```python
from build123d import *

# Parameters (mm, degrees)
SKETCH1_W           = 50
SKETCH1_H           = 70
SKETCH1_W_2         = 42
SKETCH1_H_2         = 62
BOSS_EXTRUDE2_DEPTH = 1400
SKETCH2_R           = 15
CUT_EXTRUDE1_DEPTH  = 1403.640367307


with BuildPart() as part:
    # Sketch1 → Boss-Extrude2 (new body)
    with BuildSketch(Plane.XY):
        with Locations((25, -35)):
            Rectangle(SKETCH1_W, SKETCH1_H)
        with Locations((25, -35)):
            Rectangle(SKETCH1_W_2, SKETCH1_H_2, mode=Mode.SUBTRACT)
    extrude(amount=BOSS_EXTRUDE2_DEPTH)

    # Sketch2 → Cut-Extrude1 (cut, through all)
    with BuildSketch(Plane(origin=(50, 0, 0), x_dir=(0, 0, -1), z_dir=(1, 0, 0))):
        with Locations(Location((-1050, -23, 0), (0, 0, 90))):
            Circle(SKETCH2_R)
        with Locations(Location((-200, -23, 0), (0, 0, 90))):
            Circle(SKETCH2_R)
        with Locations(Location((-810, -23, 0), (0, 0, 90))):
            Circle(SKETCH2_R)
        with Locations(Location((-360, -23, 0), (0, 0, 90))):
            Circle(SKETCH2_R)
        with BuildLine():
            Line((-1281.339745962, -30), (-1280, -30))
            ThreePointArc((-1280, -30), (-1275, -35), (-1280, -40))
            Line((-1280, -40), (-1281.339745962, -40))
            ThreePointArc((-1281.339745962, -40), (-1290, -45), (-1298.660254038, -40))
            Line((-1298.660254038, -40), (-1300, -40))
            ThreePointArc((-1300, -40), (-1305, -35), (-1300, -30))
            Line((-1300, -30), (-1298.660254038, -30))
            ThreePointArc((-1298.660254038, -30), (-1290, -25), (-1281.339745962, -30))
        make_face()
        with BuildLine():
            Line((-611.339745962, -30), (-610, -30))
            ThreePointArc((-610, -30), (-605, -35), (-610, -40))
            Line((-610, -40), (-611.339745962, -40))
            ThreePointArc((-611.339745962, -40), (-620, -45), (-628.660254038, -40))
            Line((-628.660254038, -40), (-630, -40))
            ThreePointArc((-630, -40), (-635, -35), (-630, -30))
            Line((-630, -30), (-628.660254038, -30))
            ThreePointArc((-628.660254038, -30), (-620, -25), (-611.339745962, -30))
        make_face()
    extrude(amount=-CUT_EXTRUDE1_DEPTH, mode=Mode.SUBTRACT)


solid = part.part
```
Part model, mm, in its own coordinate system. A direction names the side the tool comes from. Round coordinates to 2 decimals unless told otherwise and drop trailing zeros. Write each loop counter-clockwise with the first axis right and the second up, starting at its lowest first coordinate (ties: lowest second). Pieces come first, ordered by that corner, then holes. Notation, with made-up numbers: (73, 45.5) -> (115, 45.5) arc R25 cw to (115, 70.5) -> close; hole circle Ø3 at (55.5, 14). An arc over 180 degrees is marked (long way). Return JSON: item names as keys, results as strings. Group by question number.
Q1. Which spindle directions (+Z, -Z, +X, -X, +Y, -Y) get a long thin tool onto all of the face, cutting with end or side? Do faces 5 (the flat face through (46, -35, 690)), 6 (the flat face through (25, 0, 690)). Say none if no direction does.
Q2. Probe L1, parallel to Z at x = 2.45, y = -23; L2, parallel to X at y = -34.5, z = 1024; L3, parallel to Y at x = 44.5, z = 345.5. List the from-to ranges inside material, lowest first. Write a range as [from, to].
Q3. Mould opens along Z. For faces 1 (the cylindrical face through (48.028, -24.953, 374.872)), 2 (the flat face through (25, -4, 690)), 3 (the flat face through (3, -32, 0)), 4 (the cylindrical face through (48.028, -26.252, 795.357)) say: pulls with the +Z half, pulls with the -Z half, needs draft (parallel to the pull), parting line crosses it, or undercut.
Q4. Saw through at C-C on z = 535.5. Write the cut outline in (x, y).
Q5. Saw through at B-B on x = 36.5. Write the cut outline in (y, z).
Q6. Saw through at A-A on z = 1050. Write the cut outline in (x, y), plus the area to 3 significant figures.
Answer:
{
 "1": {"face 5": "+Z, -Z", "face 6": "+Z, -Z, +X, -X, +Y"},
 "2": {"L1": "[0, 185], [215, 345], [375, 795], [825, 1035], [1065, 1400]", "L2": "[0, 4], [46, 50]", "L3": "[-70, -66], [-4, 0]"},
 "3": {"face 1": "undercut", "face 2": "needs draft", "face 3": "pulls with the -Z half", "face 4": "undercut"},
 "4": {"outline": "(0, -70) -> (50, -70) -> (50, 0) -> (0, 0) -> close; hole (4, -66) -> (46, -66) -> (46, -4) -> (4, -4) -> close"},
 "5": {"outline": "(-70, 0) -> (-66, 0) -> (-66, 1400) -> (-70, 1400) -> close; (-4, 0) -> (0, 0) -> (0, 1400) -> (-4, 1400) -> close"},
 "6": {"outline": "(0, -70) -> (50, -70) -> (50, -38) -> (46, -38) -> (46, -66) -> (4, -66) -> (4, -38) -> (0, -38) -> close; (0, -8) -> (4, -8) -> (4, -4) -> (46, -4) -> (46, -8) -> (50, -8) -> (50, 0) -> (0, 0) -> close", "area": "656 mm2"}
}
